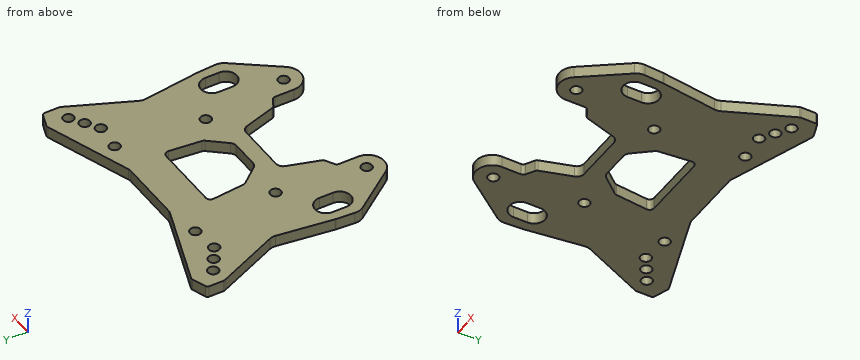
from build123d import *

# Parameters (mm, degrees)
BOSS_EXTRUDE1_DEPTH = 3.175
SKETCH2_R           = 1.4732
CUT_EXTRUDE1_DEPTH  = 66.187440595


with BuildPart() as part:
    # Sketch1 → Boss-Extrude1 (new body)
    with BuildSketch(Plane.XY):
        with BuildLine():
            Line((-8.644986321, 0), (8.644986321, 0))
            ThreePointArc((8.644986321, 0), (9.036676671, 0.033358008), (9.41708521, 0.132471226))
            Line((9.41708521, 0.132471226), (32.695027169, 8.362466532))
            ThreePointArc((32.695027169, 8.362466532), (33.037413575, 8.420565737), (33.379365385, 8.359961043))
            Line((33.379365385, 8.359961043), (37.074831276, 7.022895104))
            ThreePointArc((37.074831276, 7.022895104), (37.438600447, 6.745086623), (37.577573101, 6.308976358))
            Line((37.577573101, 6.308976358), (37.591246654, 2.336170232))
            ThreePointArc((37.591246654, 2.336170232), (37.569195736, 2.122118926), (37.502559227, 1.917512522))
            Line((37.502559227, 1.917512522), (29.896170993, -15.072175319))
            ThreePointArc((29.896170993, -15.072175319), (29.651900561, -15.913690011), (29.646955985, -16.789926606))
            Line((29.646955985, -16.789926606), (31.669948024, -31.934678241))
            ThreePointArc((31.669948024, -31.934678241), (31.684578491, -32.059980985), (31.695052571, -32.185699407))
            Line((31.695052571, -32.185699407), (32.037376325, -37.320766007))
            ThreePointArc((32.037376325, -37.320766007), (31.88963719, -38.653858534), (31.289084234, -39.853149444))
            Line((31.289084234, -39.853149444), (22.711313793, -51.345361524))
            ThreePointArc((22.711313793, -51.345361524), (17.658131065, -52.930106933), (14.566913248, -48.630055061))
            Line((14.566913248, -48.630055061), (14.5796, -43.389351757))
            ThreePointArc((14.5796, -43.389351757), (14.441970337, -42.876278099), (14.064222513, -42.502790371))
            Line((14.064222513, -42.502790371), (11.798676805, -41.21993315))
            ThreePointArc((11.798676805, -41.21993315), (11.507576341, -40.972569428), (11.3284, -40.635191111))
            Line((11.3284, -40.635191111), (8.709628272, -32.14188038))
            ThreePointArc((8.709628272, -32.14188038), (7.974572044, -31.105726569), (6.767835591, -30.7086))
            Line((6.767835591, -30.7086), (-6.767835591, -30.7086))
            ThreePointArc((-6.767835591, -30.7086), (-7.974572044, -31.105726569), (-8.709628272, -32.14188038))
            Line((-8.709628272, -32.14188038), (-11.3284, -40.635191111))
            ThreePointArc((-11.3284, -40.635191111), (-11.507576341, -40.972569428), (-11.798676805, -41.21993315))
            Line((-11.798676805, -41.21993315), (-14.064222513, -42.502790371))
            ThreePointArc((-14.064222513, -42.502790371), (-14.441970337, -42.876278099), (-14.5796, -43.389351757))
            Line((-14.5796, -43.389351757), (-14.566913248, -48.630055061))
            ThreePointArc((-14.566913248, -48.630055061), (-17.658131065, -52.930106933), (-22.711313793, -51.345361524))
            Line((-22.711313793, -51.345361524), (-31.289084234, -39.853149444))
            ThreePointArc((-31.289084234, -39.853149444), (-31.88963719, -38.653858534), (-32.037376325, -37.320766007))
            Line((-32.037376325, -37.320766007), (-31.695052571, -32.185699407))
            ThreePointArc((-31.695052571, -32.185699407), (-31.684578491, -32.059980985), (-31.669948024, -31.934678241))
            Line((-31.669948024, -31.934678241), (-29.646955985, -16.789926606))
            ThreePointArc((-29.646955985, -16.789926606), (-29.651900561, -15.913690011), (-29.896170993, -15.072175319))
            Line((-29.896170993, -15.072175319), (-37.502559227, 1.917512522))
            ThreePointArc((-37.502559227, 1.917512522), (-37.569195736, 2.122118926), (-37.591246654, 2.336170232))
            Line((-37.591246654, 2.336170232), (-37.577573101, 6.308976358))
            ThreePointArc((-37.577573101, 6.308976358), (-37.438600447, 6.745086623), (-37.074831276, 7.022895104))
            Line((-37.074831276, 7.022895104), (-33.379365385, 8.359961043))
            ThreePointArc((-33.379365385, 8.359961043), (-33.037413575, 8.420565737), (-32.695027169, 8.362466532))
            Line((-32.695027169, 8.362466532), (-9.41708521, 0.132471226))
            ThreePointArc((-9.41708521, 0.132471226), (-9.036676671, 0.033358008), (-8.644986321, 0))
        make_face()
        with BuildLine():
            Line((-3.720594556, -26.2128), (3.720594556, -26.2128))
            ThreePointArc((3.720594556, -26.2128), (4.583419353, -26.020516655), (5.282950018, -25.480057253))
            Line((5.282950018, -25.480057253), (9.168332687, -20.807888736))
            ThreePointArc((9.168332687, -20.807888736), (9.363351592, -20.486269793), (9.455616357, -20.121635275))
            Line((9.455616357, -20.121635275), (10.325877008, -11.377982322))
            ThreePointArc((10.325877008, -11.377982322), (10.003567813, -10.39980442), (9.062121174, -9.9822))
            Line((9.062121174, -9.9822), (-9.062121174, -9.9822))
            ThreePointArc((-9.062121174, -9.9822), (-10.003567813, -10.39980442), (-10.325877008, -11.377982322))
            Line((-10.325877008, -11.377982322), (-9.455616357, -20.121635275))
            ThreePointArc((-9.455616357, -20.121635275), (-9.363351592, -20.486269793), (-9.168332687, -20.807888736))
            Line((-9.168332687, -20.807888736), (-5.282950018, -25.480057253))
            ThreePointArc((-5.282950018, -25.480057253), (-4.583419353, -26.020516655), (-3.720594556, -26.2128))
        make_face(mode=Mode.SUBTRACT)
    extrude(amount=BOSS_EXTRUDE1_DEPTH)

    # Sketch2 → Cut-Extrude1 (cut, through all)
    with BuildSketch(Plane.XY.offset(3.175)):
        with Locations((33.0454, 2.451609921)):
            Circle(SKETCH2_R)
        with Locations((29.4513, 0.151296675)):
            Circle(SKETCH2_R)
        with Locations((25.8572, -2.149016571)):
            Circle(SKETCH2_R)
        with Locations((18.4277, -1.450311364)):
            Circle(SKETCH2_R)
        with Locations((15.9258, -25.093922391)):
            Circle(SKETCH2_R)
        with Locations((18.9357, -48.395328507)):
            Circle(SKETCH2_R)
        with Locations(Location((-18.9357, -48.395328507, 0), (0, 0, 180))):
            Circle(SKETCH2_R)
        with Locations(Location((-15.9258, -25.093922391, 0), (0, 0, 180))):
            Circle(SKETCH2_R)
        with Locations(Location((-18.4277, -1.450311364, 0), (0, 0, 180))):
            Circle(SKETCH2_R)
        with Locations(Location((-25.8572, -2.149016571, 0), (0, 0, 180))):
            Circle(SKETCH2_R)
        with Locations(Location((-29.4513, 0.151296675, 0), (0, 0, 180))):
            Circle(SKETCH2_R)
        with Locations(Location((-33.0454, 2.451609921, 0), (0, 0, 180))):
            Circle(SKETCH2_R)
        with BuildLine():
            Line((29.083, -32.893), (29.083, -36.703))
            ThreePointArc((29.083, -36.703), (26.035, -39.751), (22.987, -36.703))
            Line((22.987, -36.703), (22.987, -32.893))
            ThreePointArc((22.987, -32.893), (26.035, -29.845), (29.083, -32.893))
        make_face()
        with BuildLine():
            Line((-29.083, -32.893), (-29.083, -36.703))
            ThreePointArc((-29.083, -36.703), (-26.035, -39.751), (-22.987, -36.703))
            Line((-22.987, -36.703), (-22.987, -32.893))
            ThreePointArc((-22.987, -32.893), (-26.035, -29.845), (-29.083, -32.893))
        make_face()
    extrude(amount=-CUT_EXTRUDE1_DEPTH, mode=Mode.SUBTRACT)


solid = part.part
The model under review builds one solid part; all positions refer to its coordinate system, in mm. Give positions to 0.01 mm unless a question says otherwise; leave off trailing zeros. Write each loop counter-clockwise with the first axis right and the second up, starting at its lowest first coordinate (ties: lowest second). Pieces come first, ordered by that corner, then holes. Notation, with made-up numbers: M -3,20.5 L 50,20.5 A27 cw 50,57.5 Z; hole C 13,26 d5. An arc over 180 degrees is marked long. One line per question, with ' | ' between items. Start each with the question number.
Item 1: We need section C-C on y = -8. Write out the cut boundary in (x, z) (3 decimals), plus the area to 3 significant figures.
Item 2: For pin 1 (4.5 mm diameter, centred on x = 33.05, y = 2.45, fed in from +Z) (3 decimals); pin 2 (1.6 mm diameter, centred on y = -35, z = 2.5, fed in from -X), all flat-tipped, find the tip position at first contact; note any pin that passes through.
Item 3: We need section B-B on z = 1. Give the number of separate pieces and of enclosed holes in the cut face, plus the area to 3 significant figures.
Item 4: We need section A-A on x = -2. Write out the cut boundary in (y, z) (3 decimals), plus the area to 3 significant figures.
Item 5: Wall thickness on line 1 (Y direction, x = 19.5, z = 2.1); line 2 (Y direction, x = 25, z = 2.45); line 3 (Y direction, x = -3.5, z = 0.45): over which ranges is each line inside the solid? List them lowest first. Write a range as from..to.
Results found:
1) outline: M -33.062,0 L 33.062,0 L 33.062,3.175 L -33.062,3.175 Z | area: 210 mm2
2) pin 1: stops at z = 3.175 | pin 2: stops at x = -31.94
3) separate pieces: 1 | enclosed holes: 15 | area: 2,470 mm2
4) outline: M -30.709,0 L -26.213,0 L -26.213,3.175 L -30.709,3.175 Z; M -9.982,0 L 0,0 L 0,3.175 L -9.982,3.175 Z | area: 46.0 mm2
5) line 1: y = -53.14..-49.76, -47.03..-2.46, -0.44..3.7 | line 2: y = -48.28..-39.57, -30.03..-3.35, -0.95..5.64 | line 3: y = -30.71..-26.21, -9.98..0
